```python
from build123d import *

# Parameters (mm, degrees)
SKETCH1_R               = 1.9
BOSS_EXTRUDE1_DEPTH     = 6.05
CUT_EXTRUDE1_DEPTH      = 19
CUT_EXTRUDE1_DEPTH_BACK = 21
SKETCH2_R               = 2.2
CHAMFER2_SIZE           = 1
CUT_EXTRUDE2_DEPTH      = 10
CUT_EXTRUDE2_DEPTH_BACK = 10


with BuildPart() as part:
    # Sketch1 → Boss-Extrude1 (new body)
    with BuildSketch(Plane(origin=(0, 0, 0), x_dir=(1, 0, 0), z_dir=(0, 1, 0))):
        with BuildLine():
            Line((-0.061383878, 3.899516896), (6.321978872, 4))
            Line((6.321978872, 4), (13.678021128, 4))
            Line((13.678021128, 4), (13.678021128, -4))
            Line((13.678021128, -4), (6.321978872, -4))
            Line((6.321978872, -4), (-0.061383878, -3.899516896))
            ThreePointArc((-0.061383878, -3.899516896), (-3.9, 0), (-0.061383878, 3.899516896))
        make_face()
        with Locations(Location((0, 0, 0), (0, 0, 270))):
            Circle(SKETCH1_R, mode=Mode.SUBTRACT)
    extrude(amount=BOSS_EXTRUDE1_DEPTH)

    # Sketch2 → Cut-Extrude1 (cut, two sides: drawn at the far end of the back side and taken through both)
    with BuildSketch(Plane.XY.offset(-CUT_EXTRUDE1_DEPTH_BACK)):
        with Locations(Location((10, 3.025, 0), (0, 0, 180))):
            Circle(SKETCH2_R)
    extrude(amount=CUT_EXTRUDE1_DEPTH + CUT_EXTRUDE1_DEPTH_BACK, mode=Mode.SUBTRACT)

    # Chamfer2
    chamfer2_edges = [part.edges().sort_by_distance(p)[0] for p in [
        (13.678021128, 3.025, -4),
        (13.678021128, 3.025, 4),
    ]]
    chamfer(chamfer2_edges, length=CHAMFER2_SIZE)

    # Sketch3 → Cut-Extrude2 (cut, two sides: drawn at the far end of the back side and taken through both)
    with BuildSketch(Plane.XY.offset(-CUT_EXTRUDE2_DEPTH_BACK)):
        Polygon((-3.9, 3.025), (3.241860159, 3.025), (6.321978872, 6.05), (-3.9, 6.05), align=None)
    extrude(amount=CUT_EXTRUDE2_DEPTH + CUT_EXTRUDE2_DEPTH_BACK, mode=Mode.SUBTRACT)


solid = part.part
```
Work out the finished part from the listing and answer in its coordinate system (mm). A direction names the side the tool comes from. Give positions to 0.01 mm unless a question says otherwise; leave off trailing zeros. Loops run counter-clockwise (first coordinate to the right, second up) from the corner with the lowest first, then second, coordinate; pieces in that order, holes last. Notation, with made-up numbers: (-1.75, -25.5) -> (53.25, -25.5) arc R16 ccw to (53.25, 3.5) -> close; hole circle Ø11 at (16, -20). An arc over 180 degrees is marked (long way). Put each result on its own line as item: value. Start each with the question number.
Item 1: The part is cut by section D-D (z = 2.5). Give the vertices of the cut face in (x, y) (3 decimals), then the cut area to 3 significant figures.
Item 2: Each of these flat-tipped pins is pushed along its axis until it touches: P1, Ø3.5, axis at x = 10, y = 3.025, coming from the +Z side; P2, Ø1.5, axis at y = 1.5, z = 2.5, coming from the -X side; P3, Ø1, axis at x = 4.5, y = 4, coming from the +Z side. Where does it stop, or does it pass through?
Item 3: The part is cut by section A-A (z = 0). Give the vertices of the cut face in (x, y) (3 decimals), then the cut area to 3 significant figures.
Item 4: The mould has two halves that part along Z. Classify faces 3 (the face through (8.1, 1.6, 4)), 4 (the face through (-0.728, 1.491, 1.755)), 5 (the face through (13.678, 3, 0)): released by +Z, released by -Z, zero draft, split by the parting line, or undercut.
Item 5: The part is cut by section B-B (y = 1.5). Give the vertices of the cut face in (x, z), then the cut area to 3 significant figures.
Item 6: The part is cut by section C-C (x = 10). Give the vertices of the cut face in (y, z) (3 decimals).
Item 7: Find the intervals of material crossed by L1, parallel to Y at x = 10, z = 2 (3 decimals); L2, parallel to X at y = 2, z = -0.5; L3, parallel to Y at x = -2.75, z = 2.5 (3 decimals), in increasing order. Write a range as [from, to].
Item 8: Which of the six approach directions +Z, -Z, +X, -X, +Y, -Y give full straight-line access (tool end or side, diameter ignored) to faces 1 (the face through (-3.9, 1.5, 0.1)), 2 (the face through (-1, 3.025, -2))?
Answers below:
1. outline: (-2.993, 0) -> (13.678, 0) -> (13.678, 6.05) -> (6.322, 6.05) -> (3.242, 3.025) -> (-2.993, 3.025) -> close; hole circle Ø4.4 at (10, 3.025)
1. area: 62.1 mm2
2. P1: through
2. P2: x = -3.49
2. P3: z = 3.98
3. outline: (-3.9, 0) -> (-1.9, 0) -> (-1.9, 3.025) -> (-3.9, 3.025) -> close; (1.9, 0) -> (13.678, 0) -> (13.678, 6.05) -> (6.322, 6.05) -> (3.242, 3.025) -> (1.9, 3.025) -> close; hole circle Ø4.4 at (10, 3.025)
3. area: 53.4 mm2
4. face 3: released by +Z
4. face 4: undercut
4. face 5: zero draft
5. outline: (-0.06, -3.9) -> (6.32, -4) -> (8.41, -4) -> (8.41, 4) -> (6.32, 4) -> (-0.06, 3.9) arc R3.9 ccw to start; (11.59, -4) -> (12.68, -4) -> (13.68, -3) -> (13.68, 3) -> (12.68, 4) -> (11.59, 4) -> close; hole circle Ø3.8 at (0, 0)
5. area: 95.0 mm2
6. outline: (0, -4) -> (0.825, -4) -> (0.825, 4) -> (0, 4) -> close; (5.225, -4) -> (6.05, -4) -> (6.05, 4) -> (5.225, 4) -> close
7. L1: [0, 0.825], [5.225, 6.05]
7. L2: [-3.87, -1.83], [1.83, 8.05], [11.95, 13.68]
7. L3: [0, 3.025]
8. face 1: -X, +Y, -Y
8. face 2: +Z, -Z, -X, +Y
